Geometry: see drawing. Coordinates: mm, zero at the bounding-box minimum. Round coordinates to 2 decimals unless told otherwise and drop trailing zeros. Write each loop counter-clockwise with the first axis right and the second up, starting at its lowest first coordinate (ties: lowest second). Pieces come first, ordered by that corner, then holes. Notation, with made-up numbers: M 23,-33.5 L 75,-33.5 A15 ccw 75,-4.5 Z; hole C 63,1.25 d10. An arc over 180 degrees is marked long. Use one line per item in the form item = value. Start each with the question number.
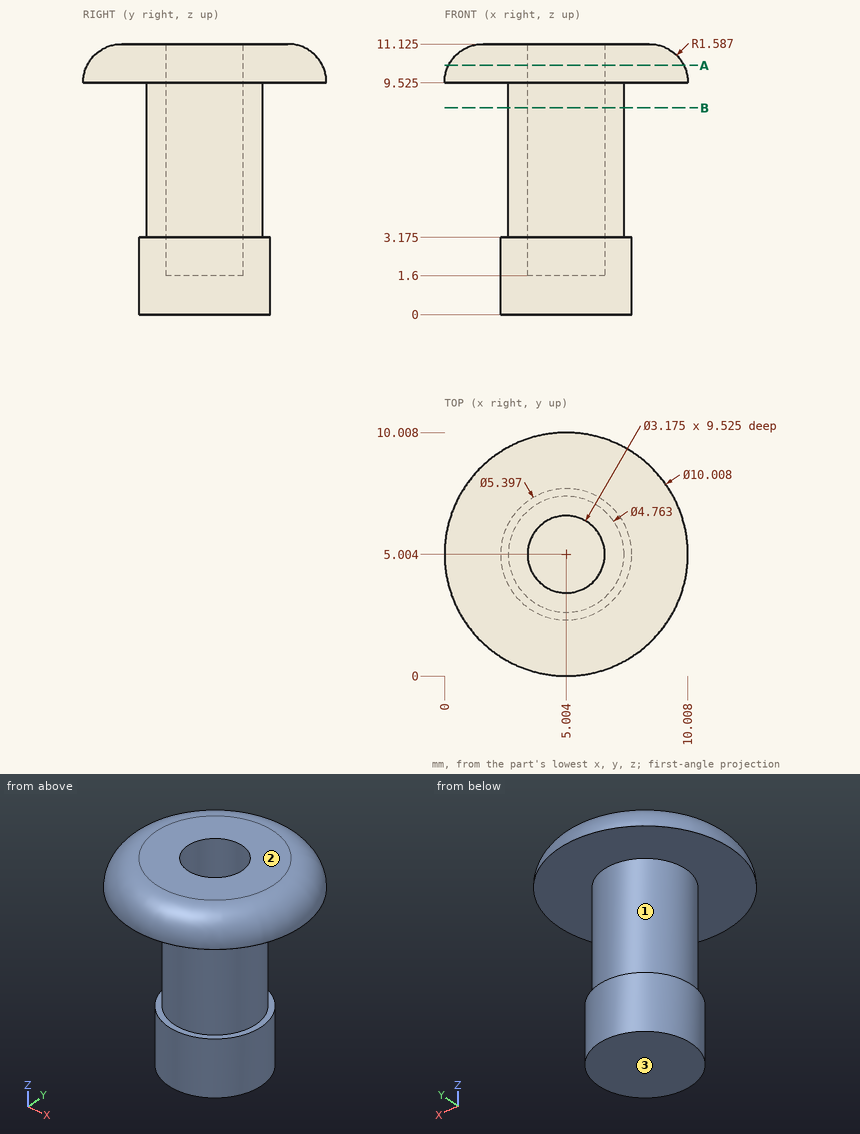
Item 1: Cut plane B-B (z = 8.5). Output: boundary loops of the cut face in (x, y) (1 decimal).
Item 2: Ray query, line 1 (Z direction, x = 2.75, y = 4) (1 decimal); line 2 (Y direction, x = 5, z = 4.5) (1 decimal); line 3 (Y direction, x = 4, z = 10) (1 decimal). Return the intervals inside material, ascending. Write a range as from..to.
Item 3: First-contact query: pin 1 (2 mm diameter, centred on x = 2, z = 7.5, fed in from -Y) (1 decimal); pin 2 (6 mm diameter, centred on x = 6, z = 2, fed in from +Y); pin 3 (1 mm diameter, centred on x = 5, y = 5.5, fed in from +Z). Flat tips, straight axial feed; report the tip coordinate or a pass-through.
Item 4: Draft query along Z for the marked faces 1, 2 and 3. Return one class per face: +Z half, -Z half, draft (parallel to the pull), parting line (faces both ways), or undercut.
Item 5: Cut plane A-A (z = 10.25). Output: boundary loops of the cut face in (x, y) (1 decimal).
Final values:
q1.outline = C 5,5 d4.8; hole C 5,5 d3.2
q2.line_1 = 0..3.2, 9.5..11.1
q2.line_2 = 2.6..3.4, 6.6..7.4
q2.line_3 = 0.2..3.8, 6.2..9.8
q3.pin_1 = 3.7
q3.pin_2 = 7.7
q3.pin_3 = 1.6
q4.face_1 = undercut
q4.face_2 = +Z half
q4.face_3 = -Z half
q5.outline = C 5,5 d9.7; hole C 5,5 d3.2
